Here's how the part is built. I have some questions about the finished solid (model axes, mm). Round coordinates to 2 decimals unless told otherwise and drop trailing zeros. Write each loop counter-clockwise with the first axis right and the second up, starting at its lowest first coordinate (ties: lowest second). Pieces come first, ordered by that corner, then holes. Notation, with made-up numbers: (64.25, 5.25) -> (106.25, 5.25) arc R7 cw to (106.25, 17.25) -> close; hole circle Ø7 at (24, 16.25). An arc over 180 degrees is marked (long way). Put each result on its own line as item: value. Start each with the question number.
1. We'd pull the mould along Z, two halves only. Please class faces 1 (the face through (-1, 1, 6)), 2 (the face through (0, 0, -8)), 3 (the face through (-4.88, 37.18, 4.99)): +Z half, -Z half, draft (parallel to the pull), parting line (faces both ways), or undercut.
2. Suppose I cut it at C-C (z = 1.5). Please give me the cut outline in (x, y).
3. Suppose I cut it at A-A (y = 0). Please give me the cut outline in (x, z), then the cut area to 3 significant figures.
4. I need wall thicknesses on probe 1 along Z at (x, y) = (-17, 15.5); probe 2 along Z at (x, y) = (-27.5, 14); probe 3 along Y at (x, z) = (-17.5, 4.75). Which ranges of each line are inside material? Lowest first, please. Write a range as from..to.
5. For pin 1 (8 mm diameter, centred on y = -24.5, z = -3.5, fed in from +X); pin 2 (2 mm diameter, centred on y = -1, z = -1.5, fed in from -X); pin 3 (3 mm diameter, centred on y = -4, z = -2, fed in from -X); pin 4 (1.5 mm diameter, centred on y = -10, z = 3.5, fed in from +X), each with a flat end and sliding along its axis, tell me the tip position at first contact or that it passes through.
```python
from build123d import *

# Parameters (mm, degrees)
F0_R     = 37.5
F1_DEPTH = 6
F2_SIZE2 = 24
F2_SIZE  = 4
F3_R     = 10
F4_DEPTH = 8
F5_SIZE  = 1


with BuildPart() as f1:
    # F0 (on Top) → F1 (new body)
    with BuildSketch(Plane.XY):
        Circle(F0_R)
    extrude(amount=F1_DEPTH)

    # F2
    f2_edges = [f1.edges().sort_by_distance(p)[0] for p in [
        (-37.5, 0, 0),
    ]]
    chamfer(f2_edges, length=F2_SIZE, length2=F2_SIZE2)

    # F3 (on face) → F4 (join)
    with BuildSketch(Plane(origin=(0, 0, 0), x_dir=(1, 0, 0), z_dir=(0, 0, -1))):
        Circle(F3_R)
    extrude(amount=F4_DEPTH)

    # F5
    f5_edges = [f1.edges().sort_by_distance(p)[0] for p in [
        (-10, 0, -8),
    ]]
    chamfer(f5_edges, length=F5_SIZE)


solid = f1.part
```
Verdict:
1. face 1: +Z half
1. face 2: -Z half
1. face 3: draft
2. outline: circle Ø45 at (0, 0)
3. outline: (-37.5, 4) -> (-13.5, 0) -> (-10, 0) -> (-10, -7) -> (-9, -8) -> (9, -8) -> (10, -7) -> (10, 0) -> (13.5, 0) -> (37.5, 4) -> (37.5, 6) -> (-37.5, 6) -> close
3. area: 513 mm^2
4. probe 1: z = 1.58..6
4. probe 2: z = 2.89..6
4. probe 3: y = -33.17..33.17
5. pin 1: passes through
5. pin 2: stops at x = -10
5. pin 3: stops at x = -9.68
5. pin 4: stops at x = 36.29
